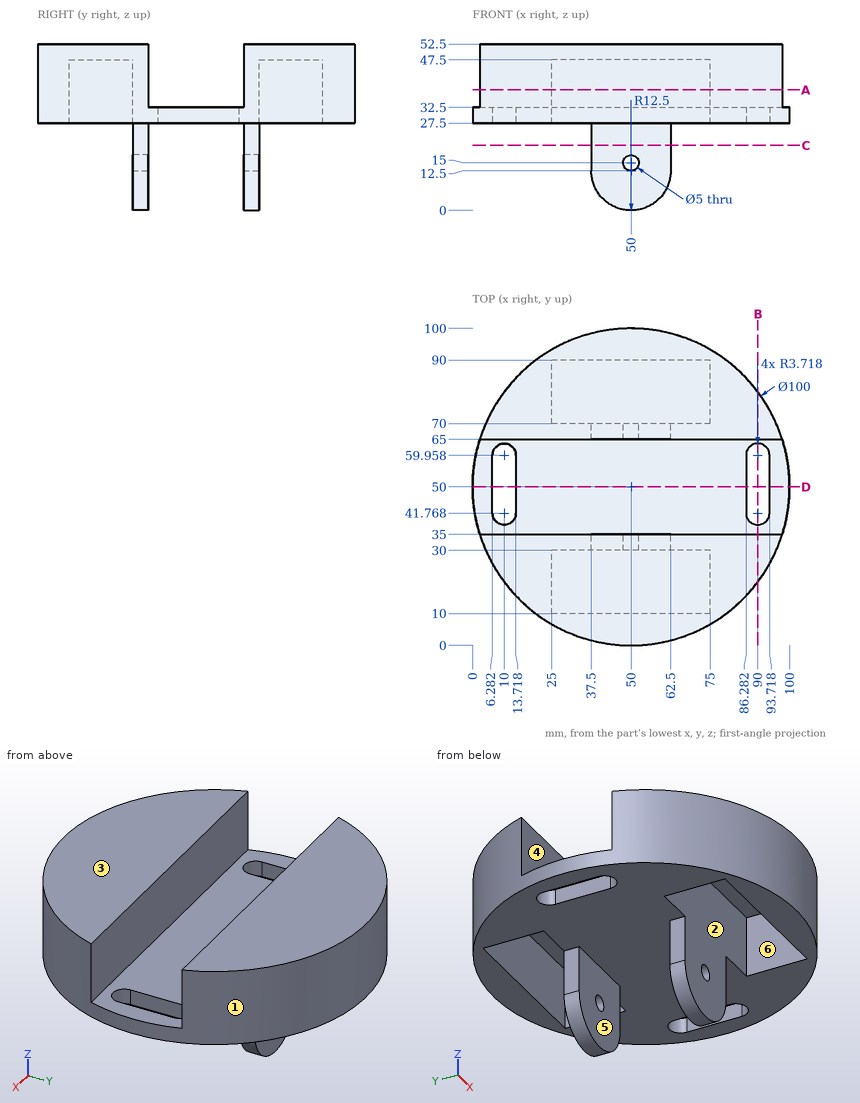
The drawing under review shows one solid part. Ordinate dimensions are in mm from its lowest x, y, z. A direction names the side the tool comes from. Round coordinates to 2 decimals unless told otherwise and drop trailing zeros. Loops run counter-clockwise (first coordinate to the right, second up) from the corner with the lowest first, then second, coordinate; pieces in that order, holes last. Notation, with made-up numbers: M 19.25,43 L 30.25,43 A28 ccw 30.25,80 Z; hole C 67,24.25 d1. An arc over 180 degrees is marked long. Answer as CSV lines item,"result". Start each with the question number.
Item 1: Consider section B-B (x = 90). Write out the cut boundary in (y, z).
Item 2: Mouldability with a two-part tool opening along X and no side actions: class the marked faces 1, 2 and 3 as released by +X, released by -X, zero draft, split by the parting line, or undercut.
Item 3: Consider section A-A (z = 38). Write out the cut boundary in (x, y).
Item 4: For the marked faces 4, 5 and 6, list the 3-axis set-ups (+Z, -Z, +X, -X, +Y, -Y) from which the entire face can be reached by the end or side of a thin tool; tool diameter is ignored.
Item 5: Consider section D-D (y = 50). Write out the cut boundary in (x, z).
Item 6: Wall thickness on line 1 (Y direction, x = 20, z = 42); line 2 (Y direction, x = 40.5, z = 19.5); line 3 (X direction, y = 66.6, z = 15): over which ranges is each line inside the solid? List them lowest first. Write a range as [from, to].
Item 7: Consider section C-C (z = 20.5). Write out the cut boundary in (x, y), then the cut area to 3 significant figures.
Item 8: Insertion check: P1, Ø5, axis at x = 59, z = 12, coming from the +Y side; P2, Ø4, axis at y = 66.5, z = 16.5, coming from the +X side; P3, Ø12, axis at x = 72, z = 36.5, coming from the +Y side; P4, Ø16, axis at x = 53, y = 76.5, coming from the -Z side. Each pin has a flat end and moves straight along its axis. Give the tip position at first contact, or say it passes through.
Answer:
1,outline,"M 20,27.5 L 38.05,27.5 L 38.05,32.5 L 35,32.5 L 35,52.5 L 20,52.5 Z; M 63.68,27.5 L 80,27.5 L 80,52.5 L 65,52.5 L 65,32.5 L 63.68,32.5 Z"
2,face 1,"split by the parting line"
2,face 2,"undercut"
2,face 3,"zero draft"
3,outline,"M 2.3,35 A50 ccw 97.7,35 Z; M 2.3,65 L 97.7,65 A50 ccw Z; hole M 25,10 L 75,10 L 75,30 L 25,30 Z; hole M 25,70 L 75,70 L 75,90 L 25,90 Z"
4,face 4,"+Z, +X, -X"
4,face 5,"-Z, +X, -X"
4,face 6,"-Z"
5,outline,"M 0,27.5 L 6.28,27.5 L 6.28,32.5 L 0,32.5 Z; M 13.72,27.5 L 86.28,27.5 L 86.28,32.5 L 13.72,32.5 Z; M 93.72,27.5 L 100,27.5 L 100,32.5 L 93.72,32.5 Z"
6,line 1,"y = [10, 35], [65, 90]"
6,line 2,"y = [30, 35], [65, 70]"
6,line 3,"x = [37.5, 47.5], [52.5, 62.5]"
7,outline,"M 37.5,30 L 62.5,30 L 62.5,35 L 37.5,35 Z; M 37.5,65 L 62.5,65 L 62.5,70 L 37.5,70 Z"
7,area,"250 mm^2"
8,P1,"stops at y = 70"
8,P2,"stops at x = 62.5"
8,P3,"stops at y = 97.37"
8,P4,"stops at z = 0"
